Geometry: final body of the model. Coordinates: model frame, mm. Face numbers are marked on the shaded views. A direction names the side the tool comes from. Round coordinates to 2 decimals unless told otherwise and drop trailing zeros. Order: outer loops, then holes, each group sorted by start corner. A loop starts at its lowest first (then second) coordinate and runs counter-clockwise, first axis right, second up. Notation, with made-up numbers: M 61.25,56.5 L 98.25,56.5 A26 ccw 98.25,93.5 Z; hole C 66.25,52 d4. An arc over 180 degrees is marked long. Return JSON: item names as keys, results as strings. Group by question number.
Q1. Mould query, pull axis Z, two halves, no side actions, for the marked faces 1, 2 and 3. Classes: released by +Z, released by -Z, zero draft, split by the parting line, or undercut.
Q2. Contact query for flat-ended pins moving along their axis: pin 1 (4.5 mm diameter, centred on y = 9, z = 6.5, fed in from +X); pin 2 (3.5 mm diameter, centred on y = 2, z = 1.5, fed in from +X); pin 3 (1.6 mm diameter, centred on x = 3, z = 5.5, fed in from -Y). Output: stop coordinate, or through.
Q3. Cut plane A-A on y = 14.7. Output: boundary loops of the cut face in (x, z), and give its area (3 significant figures).
Q4. Cut plane D-D on z = 7. Output: boundary loops of the cut face in (x, y), and give its area (3 significant figures).
Q5. Access query for the marked faces 4, 5 and 6. Directions: +Z, -Z, +X, -X, +Y, -Y. A direction counts if a zero-diameter tool reaches every point of the face in a straight line with its end or side. Return the directions, or none.
Q6. Cut plane B-B on z = 5.5. Output: boundary loops of the cut face in (x, y).
Q7. Cut plane C-C on x = 2. Output: boundary loops of the cut face in (y, z), and give its area (3 significant figures).
Q8. Ray query, probe 1 along Y at (x, z) = (2.75, 5.5); probe 2 along X at (y, z) = (16.75, 4); probe 3 along Y at (x, z) = (1.15, 5.5). Return the intervals inside material, ascending.
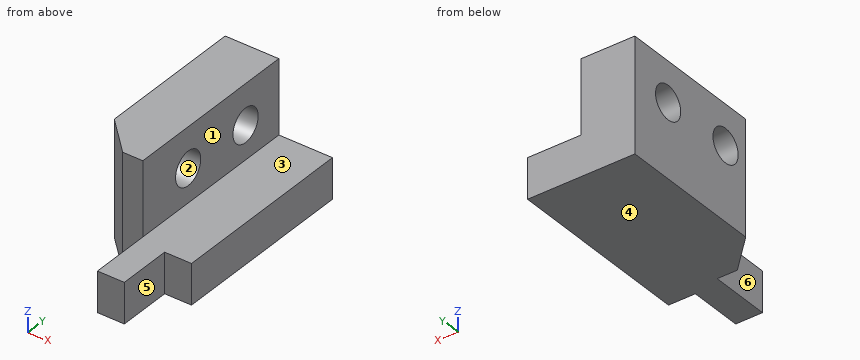
```python
from build123d import *

# Parameters (mm, degrees)
SKETCH_1_W          = 8
SKETCH_1_H          = 18
EXTRUDE_1_DEPTH     = 8.5
SKETCH_2_W          = 4
SKETCH_2_H          = 5.5
CUT_EXTRUDE_1_DEPTH = 22.453437953
HOLE_WIZARD_M3_1_D  = 2.5
SKETCH_5_W          = 5.5
SKETCH_5_H          = 4
CUT_EXTRUDE_2_DEPTH = 8.5
SKETCH_6_W          = 2
SKETCH_6_H          = 4
CUT_EXTRUDE_3_DEPTH = 21.451161336
SKETCH_7_W          = 4
SKETCH_7_H          = 4.5
CUT_EXTRUDE_4_DEPTH = 22.453437953
CHAMFER_1_SIZE      = 2.5


with BuildPart() as part:
    # 草图1 → 凸台-拉伸1 (new body)
    with BuildSketch(Plane.XY):
        with Locations((4, 9)):
            Rectangle(SKETCH_1_W, SKETCH_1_H)
    extrude(amount=EXTRUDE_1_DEPTH)

    # 草图2 → 切除-拉伸1 (cut, through all)
    with BuildSketch(Plane(origin=(0, 18, 0), x_dir=(1, 0, 0), z_dir=(0, 1, 0))):
        with Locations((6, -5.75)):
            Rectangle(SKETCH_2_W, SKETCH_2_H)
    extrude(amount=-CUT_EXTRUDE_1_DEPTH, mode=Mode.SUBTRACT)

    # M3 螺纹孔1 (through all)
    with Locations(Plane.ZY):
        with Locations((5.5, 14.7), (5.5, 9)):
            Hole(HOLE_WIZARD_M3_1_D / 2)

    # 草图5 → 切除-拉伸2 (cut)
    with BuildSketch(Plane(origin=(4, 0, 0), x_dir=(0, 0, -1), z_dir=(1, 0, 0))):
        with Locations((-5.75, 2)):
            Rectangle(SKETCH_5_W, SKETCH_5_H)
    extrude(amount=-CUT_EXTRUDE_2_DEPTH, mode=Mode.SUBTRACT)

    # 草图6 → 切除-拉伸3 (cut, through all)
    with BuildSketch(Plane.XY.offset(3)):
        with Locations((7, 2)):
            Rectangle(SKETCH_6_W, SKETCH_6_H)
    extrude(amount=-CUT_EXTRUDE_3_DEPTH, mode=Mode.SUBTRACT)

    # 草图7 → 切除-拉伸4 (cut, through all)
    with BuildSketch(Plane(origin=(0, 0, 0), x_dir=(-1, 0, 0), z_dir=(0, 0, -1))):
        with Locations((-2, 2.25)):
            Rectangle(SKETCH_7_W, SKETCH_7_H)
    extrude(amount=-CUT_EXTRUDE_4_DEPTH, mode=Mode.SUBTRACT)

    # 倒角1
    chamfer_1_edges = [part.edges().sort_by_distance(p)[0] for p in [
        (0, 4.5, 4.25),
    ]]
    chamfer(chamfer_1_edges, length=CHAMFER_1_SIZE)


solid = part.part
```
Result sheet:
{
 "1": {"face 1": "zero draft", "face 2": "undercut", "face 3": "released by +Z"},
 "2": {"pin 1": "stops at x = 4", "pin 2": "stops at x = 6", "pin 3": "stops at y = 4.5"},
 "3": {"outline": "M 0,0 L 8,0 L 8,3 L 4,3 L 4,4.25 L 0,4.25 Z; M 0,6.75 L 4,6.75 L 4,8.5 L 0,8.5 Z", "area": "36.0 mm²"},
 "4": {"outline": "M 0,7 L 2.5,4.5 L 4,4.5 L 4,18 L 0,18 Z", "area": "50.9 mm²"},
 "5": {"face 4": "-Z, +X, -X, +Y, -Y", "face 5": "+Z, -Z, +X, -Y", "face 6": "+Z, -Z, -X, -Y"},
 "6": {"outline": "M 0,7 L 2.5,4.5 L 4,4.5 L 4,7.75 L 0,7.75 Z; M 0,10.25 L 4,10.25 L 4,13.45 L 0,13.45 Z; M 0,15.95 L 4,15.95 L 4,18 L 0,18 Z"},
 "7": {"outline": "M 5,0 L 18,0 L 18,8.5 L 5,8.5 Z; hole C 9,5.5 d2.5; hole C 14.7,5.5 d2.5", "area": "101 mm²"},
 "8": {"probe 1": "y = 4.5 to 7.75, 10.25 to 13.45, 15.95 to 18", "probe 2": "x = 0 to 4", "probe 3": "y = 5.85 to 7.75, 10.25 to 13.45, 15.95 to 18"}
}
